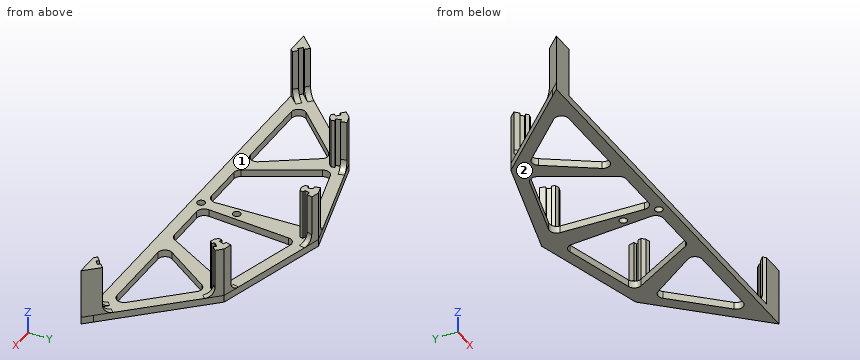
```python
from build123d import *

# Parameters (mm, degrees)
BOSS_EXTRUDE1_DEPTH = 3
BOSS_EXTRUDE2_DEPTH = 21
SKETCH3_R           = 1.642484664
CUT_EXTRUDE1_DEPTH  = 101.008681907
FILLET3_R           = 4
FILLET4_R           = 4


with BuildPart() as part:
    # Sketch1 → Boss-Extrude1 (new body)
    with BuildSketch(Plane.XY):
        Polygon((0, 46.774719198), (48.18152266, 33.412800394), (82.599251445, -2.855918156), (85.865371953, -6.297691035), (78.97237959, -6.297691035), (-78.97237959, -6.297691035), (-85.865371953, -6.297691035), (-82.599251445, -2.855918156), (-48.18152266, 33.412800394), align=None)
    extrude(amount=BOSS_EXTRUDE1_DEPTH)

    # Sketch2 → Boss-Extrude2 (add)
    with BuildSketch(Plane.XY.offset(3)):
        Polygon((-44.779907161, 34.356151862), (-48.18152266, 33.412800394), (-50.611414313, 30.852228864), (-48.870515822, 29.200177883), (-47.989421965, 30.128657078), (-46.393598349, 28.614277011), (-47.274692206, 27.685797816), (-46.22623914, 26.690853007), (-44.440185395, 27.186169547), (-43.164345406, 28.530624372), (-43.550610631, 29.923451777), (-44.784057611, 29.581386656), (-45.371982038, 31.701373653), (-44.138535058, 32.043438774), align=None)
        Polygon((0, 46.774719198), (-3.4016155, 45.83136773), (-2.760243397, 43.518654643), (-1.526796417, 43.860719764), (-0.93887199, 41.740732767), (-2.17231897, 41.398667646), (-1.786053745, 40.00584024), (0, 39.5105237), (1.786053745, 40.00584024), (2.17231897, 41.398667646), (0.93887199, 41.740732767), (1.526796417, 43.860719764), (2.760243397, 43.518654643), (3.4016155, 45.83136773), align=None)
        Polygon((-78.428461302, -1.947397608), (-80.169359793, -0.295346627), (-85.865371953, -6.297691035), (-76.215182645, -6.297691035), (-75.091739196, -5.113828657), (-76.832637686, -3.461777675), (-77.713731543, -4.39025687), (-79.309555159, -2.875876803), align=None)
        Polygon((48.18152266, 33.412800394), (44.779907161, 34.356151862), (44.138535058, 32.043438774), (45.371982038, 31.701373653), (44.784057611, 29.581386656), (43.550610631, 29.923451777), (43.164345406, 28.530624372), (44.440185395, 27.186169547), (46.22623914, 26.690853007), (47.274692206, 27.685797816), (46.393598349, 28.614277011), (47.989421965, 30.128657078), (48.870515822, 29.200177883), (50.611414313, 30.852228864), align=None)
        Polygon((75.091739196, -5.113828657), (76.215182645, -6.297691035), (85.865371953, -6.297691035), (80.169359793, -0.295346627), (78.428461302, -1.947397608), (79.309555159, -2.875876803), (77.713731543, -4.39025687), (76.832637686, -3.461777675), align=None)
    extrude(amount=BOSS_EXTRUDE2_DEPTH)

    # Sketch3 → Cut-Extrude1 (cut, through all)
    with BuildSketch(Plane.XY.offset(3)):
        with Locations((0, -2.554468846)):
            Circle(SKETCH3_R)
        with Locations((0, 12.445531154)):
            Circle(SKETCH3_R)
        with BuildLine():
            Line((-69.420990751, 3.767372692), (-50.828151114, 23.360137575))
            ThreePointArc((-50.828151114, 23.360137575), (-48.390560772, 24.283657942), (-46.150370534, 22.950884804))
            Line((-46.150370534, 22.950884804), (-33.182202355, 3.358119921))
            ThreePointArc((-33.182202355, 3.358119921), (-33.041187606, 0.282349963), (-35.683859821, -1.297691035))
            Line((-35.683859821, -1.297691035), (-67.244867638, -1.297691035))
            ThreePointArc((-67.244867638, -1.297691035), (-70.001241269, 0.518077396), (-69.420990751, 3.767372692))
        make_face()
        with BuildLine():
            Line((-25.543650537, 0.270832684), (-39.897767636, 26.707827652))
            ThreePointArc((-39.897767636, 26.707827652), (-40.022830858, 29.311497318), (-38.063031426, 31.030195292))
            Line((-38.063031426, 31.030195292), (-8.166425929, 39.321257781))
            ThreePointArc((-8.166425929, 39.321257781), (-5.611961803, 38.865088367), (-4.368822196, 36.58737429))
            Line((-4.368822196, 36.58737429), (-2.558453179, 2.043475626))
            ThreePointArc((-2.558453179, 2.043475626), (-3.426038324, -0.308216813), (-5.729101952, -1.297691035))
            Line((-5.729101952, -1.297691035), (-22.907199199, -1.297691035))
            ThreePointArc((-22.907199199, -1.297691035), (-24.441078457, -0.875910269), (-25.543650537, 0.270832684))
        make_face()
        with BuildLine():
            Line((5.729101952, -1.297691035), (22.907199199, -1.297691035))
            ThreePointArc((22.907199199, -1.297691035), (24.441078457, -0.875910269), (25.543650537, 0.270832684))
            Line((25.543650537, 0.270832684), (39.897767636, 26.707827652))
            ThreePointArc((39.897767636, 26.707827652), (40.022830858, 29.311497318), (38.063031426, 31.030195292))
            Line((38.063031426, 31.030195292), (8.166425929, 39.321257781))
            ThreePointArc((8.166425929, 39.321257781), (5.611961803, 38.865088367), (4.368822196, 36.58737429))
            Line((4.368822196, 36.58737429), (2.558453179, 2.043475626))
            ThreePointArc((2.558453179, 2.043475626), (3.426038324, -0.308216813), (5.729101952, -1.297691035))
        make_face()
        with BuildLine():
            Line((35.683859821, -1.297691035), (67.244867638, -1.297691035))
            ThreePointArc((67.244867638, -1.297691035), (70.001241269, 0.518077396), (69.420990751, 3.767372692))
            Line((69.420990751, 3.767372692), (50.828151114, 23.360137575))
            ThreePointArc((50.828151114, 23.360137575), (48.390560772, 24.283657942), (46.150370534, 22.950884804))
            Line((46.150370534, 22.950884804), (33.182202355, 3.358119921))
            ThreePointArc((33.182202355, 3.358119921), (33.041187606, 0.282349963), (35.683859821, -1.297691035))
        make_face()
    extrude(amount=-CUT_EXTRUDE1_DEPTH, mode=Mode.SUBTRACT)

    # Fillet3
    fillet3_edges = [part.edges().sort_by_distance(p)[0] for p in [
        (-79.298910548, -1.121372118, 3),
    ]]
    fillet(fillet3_edges, radius=FILLET3_R)

    # Fillet4
    fillet4_edges = [part.edges().sort_by_distance(p)[0] for p in [
        (79.298910548, -1.121372118, 3),
        (49.740965067, 30.026203374, 3),
        (44.459221109, 33.199795318, 3),
        (3.080929449, 44.675011187, 3),
        (-3.080929449, 44.675011187, 3),
        (-44.459221109, 33.199795318, 3),
        (-75.962188441, -4.287803166, 3),
        (-49.740965067, 30.026203374, 3),
        (75.962188441, -4.287803166, 3),
    ]]
    fillet(fillet4_edges, radius=FILLET4_R)


solid = part.part
```
Could you check a few things on this model? Use its own coordinates, in mm. Face numbers are marked on the shaded views. Round coordinates to 2 decimals unless told otherwise and drop trailing zeros. Write each loop counter-clockwise with the first axis right and the second up, starting at its lowest first coordinate (ties: lowest second). Pieces come first, ordered by that corner, then holes. Notation, with made-up numbers: M 68,-24.75 L 124,-24.75 A32 ccw 124,3.25 Z; hole C -6.75,51 d1. An arc over 180 degrees is marked long. Write each question's results on one line, items separated by ' | '. Start each with the question number.
1. Imagine slicing it at B-B on z = 15.75. Count the separate pieces of the cut face and the enclosed holes in it, and give its area (3 significant figures).
2. Imagine slicing it at C-C on x = -60.5. List the corners of the cut face in (y, z) for me, and give its area (3 significant figures).
3. I'm going to push flat-ended pins straight in: pin 1 Ø2 at (y, z) = (31.5, 21) entering from +X; pin 2 Ø12 at (x, z) = (36.5, 9.5) entering from +Y; pin 3 Ø2.5 at (x, z) = (-13.5, 2) entering from +Y; pin 4 Ø0.9 at (x, z) = (-56.5, 1.5) entering from +Y. Where does each tip first touch, or does it pass through?
4. Imagine slicing it at A-A on x = -14. List the corners of the cut face in (y, z) for me.
5. Thinking about a two-plate mould opening in X: for the marked faces 1 and 2, which applies, +X half, -X half, draft (parallel to the pull), parting line (faces both ways), or undercut?
6. I need wall thicknesses on L1, parallel to Y at x = 0, z = 1.35; L2, parallel to X at y = 13.5, z = 2; L3, parallel to Z at x = -28.5, y = -1.5. Which ranges of each line are inside material? Lowest first, please. Write a range as from..to.
Result sheet:
1) separate pieces: 5 | enclosed holes: 0 | area: 150 mm^2
2) outline: M -6.3,0 L -1.3,0 L -1.3,3 L -6.3,3 Z; M 13.17,0 L 20.43,0 L 20.43,3 L 13.17,3 Z | area: 36.8 mm^2
3) pin 1: stops at x = 50.61 | pin 2: passes through | pin 3: stops at y = 43.38 | pin 4: stops at y = 25.12
4) outline: M -6.3,0 L -1.3,0 L -1.3,3 L -6.3,3 Z; M 37.7,0 L 42.89,0 L 42.89,3 L 37.7,3 Z
5) face 1: undercut | face 2: draft
6) L1: y = -6.3..-4.2, -0.91..10.8, 14.09..46.77 | L2: x = -67.08..-60.19, -39.89..-32.73, -3.16..-1.26, 1.26..3.16, 32.73..39.89, 60.19..67.08 | L3: z = 0..3
